Autodesk Inventor part; units mm, degrees
ref_plane "YZ Plane" through (0, 0, 0) normal (1, 0, 0) x (0, 1, 0)
ref_plane "XZ Plane" through (0, 0, 0) normal (0, 1, 0) x (-1, 0, 0)
ref_plane "XY Plane" through (0, 0, 0) normal (0, 0, 1) x (1, 0, 0)
sketch "Sketch1" plane through (0, 0, 0) normal (0, 0, 1) x (1, 0, 0)
  circle A0 centre (0, 0) radius 1.2
  circle A1 centre (0, 0) radius 2.75
  line L0 (-1.75, 2.75) -> (1.75, 2.75)
  line L1 (2.75, 1.75) -> (2.75, -1.75)
  line L2 (1.75, -2.75) -> (-1.75, -2.75)
  line L3 (-2.75, -1.75) -> (-2.75, 1.75)
  arc A2 (-1.75, 2.75) -> (-2.75, 1.75) centre (-1.75, 1.75) ccw
  arc A3 (2.75, 1.75) -> (1.75, 2.75) centre (1.75, 1.75) ccw
  arc A4 (1.75, -2.75) -> (2.75, -1.75) centre (1.75, -1.75) ccw
  arc A5 (-2.75, -1.75) -> (-1.75, -2.75) centre (-1.75, -1.75) ccw
  line L4 (-2.75, 0) -> (2.75, 0)
  line L5 (2.75, 0) -> (2.75, 11.75)
  line L6 (1.75, 12.75) -> (-1.75, 12.75)
  line L7 (-2.75, 11.75) -> (-2.75, 0)
  circle A6 centre (0, 10) radius 2.75
  circle A7 centre (0, 10) radius 1.2
  arc A8 (-1.75, 12.75) -> (-2.75, 11.75) centre (-1.75, 11.75) ccw
  arc A9 (2.75, 11.75) -> (1.75, 12.75) centre (1.75, 11.75) ccw
  point P0 (-2.75, 0)
  point P1 (0, -2.75)
  point P2 (0, 0)
  point P3 (-2.75, 1.75)
  point P4 (2.75, 0)
  dimension "d0" = 2.4
  dimension "d1" = 5.5
  dimension "d2" = 1
  dimension "d3" = 1
  dimension "d4" = 1
  dimension "d11" = 2.4
  dimension "d12" = 10
  dimension "d13" = 1
  dimension "d14" = 1
extrude "Extrusion1" add sketch "Sketch1" against normal blind 5 contours L4 A0 | A0 L4
extrude "Extrusion2" add sketch "Sketch1" along normal blind 5.1 contours L4 A0 | L4 A1 A0 | A0 L4 A1 | A0 L4 | A1 L0 A3 L1 | L3 A2 L0 A1 | A1 L2 A5 L3 | L0 A2 L7 A6 L5 A3 | A6 L6 A9 L5 | A6 | L7 A8 L6 A6 | A7
extrude "Extrusion3" add sketch "Sketch1" along normal blind 7.1 contours A7
equation "\"d11\" = d0"
properties part number "rpi_base_back_3DPrint"
Work out the finished part from the listing and answer in its coordinate system (mm). A direction names the side the tool comes from. Round coordinates to 2 decimals unless told otherwise and drop trailing zeros. Write each loop counter-clockwise with the first axis right and the second up, starting at its lowest first coordinate (ties: lowest second). Pieces come first, ordered by that corner, then holes.
1) A tool of negligible diameter and unlimited length cuts with its end or side. For faces 1 (the cylindrical face through (1.97, -1.92, 2.51)), 2 (the cylindrical face through (-0.26, 11.17, 6.09)), from which of +Z, -Z, +X, -X, +Y, -Y can it reach the whole face along a straight path? Write none if from no direction.
2) A cutting plane is placed at B-B (z = 2.25). Give the vertices of the cut face in (x, y).
3) Straight lines are drawn through the part: line 1 (Z direction, x = 2.35, y = 8.5); line 2 (Y direction, x = 0.3, z = 3.75); line 3 (X direction, y = 10, z = 6.25). For each, find the intervals that lie inside material, in ascending order.
4) Given pin 1 Ø3 at (x, y) = (-2, 2) entering from +Z; pin 2 Ø2 at (x, z) = (-1.5, -2.5) entering from -Y, each flat-ended and moving along its own axis, determine where each tip first touches the part or whether it passes through.
5) A cutting plane is placed at C-C (x = -0.6). Give the vertices of the cut face in (y, z).
6) The mould has two halves that part along Z. Classify faces 3 (the flat face through (0, 10, 7.1)), 4 (the cylindrical face through (0.65, 1.01, -2.46)), 5 (the flat face through (0, 0, -5)): pulls with the +Z half, pulls with the -Z half, needs draft (parallel to the pull), parting line crosses it, or undercut.
7) A cutting plane is placed at D-D (y = 7.75). Give the vertices of the cut face in (x, z).
8) A cutting plane is placed at A-A (y = 10). Give the vertices of the cut face in (x, z), plus the area to 4 significant figures.
Completed:
1. face 1: +Z, -Z, +X, -Y
1. face 2: +Z
2. outline: (-2.75, -1.75) arc R1 ccw to (-1.75, -2.75) - (0, -2.75) arc R2.75 ccw to (2.75, 0) - (2.75, 11.75) arc R1 ccw to (1.75, 12.75) - (-1.75, 12.75) arc R1 ccw to (-2.75, 11.75) - close
3. line 1: z = 0 to 5.1
3. line 2: y = -2.73 to 12.75
3. line 3: x = -1.2 to 1.2
4. pin 1: stops at z = 5.1
4. pin 2: stops at y = -1.09
5. outline: (-2.75, 0) - (-1.04, 0) - (-1.04, -5) - (1.04, -5) - (1.04, 0) - (12.75, 0) - (12.75, 5.1) - (11.04, 5.1) - (11.04, 7.1) - (8.96, 7.1) - (8.96, 5.1) - (-2.75, 5.1) - close
6. face 3: pulls with the +Z half
6. face 4: needs draft
6. face 5: pulls with the -Z half
7. outline: (-2.75, 0) - (2.75, 0) - (2.75, 5.1) - (-2.75, 5.1) - close
8. outline: (-2.75, 0) - (2.75, 0) - (2.75, 5.1) - (1.2, 5.1) - (1.2, 7.1) - (-1.2, 7.1) - (-1.2, 5.1) - (-2.75, 5.1) - close
8. area: 32.85 mm2
